For this review, take the finished solid that the model builds, in its own axes (mm). A direction names the side the tool comes from. Give positions to 0.01 mm unless a question says otherwise; leave off trailing zeros. Loops run counter-clockwise (first coordinate to the right, second up) from the corner with the lowest first, then second, coordinate; pieces in that order, holes last. Notation, with made-up numbers: (86.5, 85) - (126.5, 85) arc R11 cw to (126.5, 105) - close; hole circle Ø2 at (63.25, 42.25). An arc over 180 degrees is marked (long way). Answer in a Markdown table with one row per item.
```python
from build123d import *

# Parameters (mm, degrees)
SKETCH1_R               = 3.175
BOSS_EXTRUDE1_DEPTH     = 9.525
CUT_EXTRUDE1_DEPTH      = 6.35
CUT_EXTRUDE2_START      = -19.05
CUT_EXTRUDE2_DEPTH      = 6.35
BOSS_EXTRUDE2_DEPTH     = 6.35
CUT_EXTRUDE5_DEPTH      = 54.858594107
CUT_EXTRUDE5_DEPTH_BACK = 54.858594107


with BuildPart() as part:
    # Sketch1 → Boss-Extrude1 (new, symmetric)
    with BuildSketch(Plane.XY):
        with BuildLine():
            Line((6.300964517, 11.912379435), (50.8, 6.35))
            Line((50.8, 6.35), (7.193167088, 6.35))
            Line((7.193167088, 6.35), (6.300964517, -0.787620565))
            ThreePointArc((6.300964517, -0.787620565), (4.202446277, -4.760456416), (0, -6.35))
            ThreePointArc((0, -6.35), (-4.760456416, -4.202446277), (-6.300964517, 0.787620565))
            ThreePointArc((-6.300964517, 0.787620565), (-4.202446277, 4.760456416), (0, 6.35))
            Line((0, 6.35), (0.781538462, 12.602307692))
            Line((0.781538462, 12.602307692), (6.300964517, 11.912379435))
        make_face()
        with Locations(Location((0, 0, 0), (0, 0, 180))):
            Circle(SKETCH1_R, mode=Mode.SUBTRACT)
    extrude(amount=BOSS_EXTRUDE1_DEPTH, both=True)

    # Sketch2 → Cut-Extrude1 (cut)
    with BuildSketch(Plane.XY.offset(9.525)):
        Polygon((7.193167088, 21.115513253), (-6.35, 21.115513253), (-6.35, 0.257727368), (-6.35, -6.35), (7.193167088, -6.35), (7.193167088, 6.35), (8.941363703, 20.335572925), align=None)
    extrude(amount=-CUT_EXTRUDE1_DEPTH, mode=Mode.SUBTRACT)

    # Sketch2<2> → Cut-Extrude2 (cut)
    with BuildSketch(Plane.XY.offset(9.525).offset(CUT_EXTRUDE2_START)):
        Polygon((7.193167088, 21.115513253), (-6.35, 21.115513253), (-6.35, 0.257727368), (-6.35, -6.35), (7.193167088, -6.35), (7.193167088, 6.35), (8.941363703, 20.335572925), align=None)
    extrude(amount=CUT_EXTRUDE2_DEPTH, mode=Mode.SUBTRACT)

    # Sketch3 → Boss-Extrude2 (add)
    with BuildSketch(Plane.XY.offset(3.175)):
        with BuildLine():
            Line((-1.905, 2.54), (-1.905, -2.54))
            ThreePointArc((-1.905, -2.54), (-3.175, 0), (-1.905, 2.54))
        make_face()
    extrude(amount=-BOSS_EXTRUDE2_DEPTH)

    # Sketch4 → Cut-Extrude5 (cut, two sides: drawn at the far end of the back side and taken through both)
    with BuildSketch(Plane.XY.offset(3.175).offset(-CUT_EXTRUDE5_DEPTH_BACK)):
        with BuildLine():
            Line((0.787620565, 6.300964517), (1.563076923, 12.504615385))
            Line((1.563076923, 12.504615385), (-1.51572631, 12.889465789))
            Line((-1.51572631, 12.889465789), (-2.391608705, 5.882406634))
            ThreePointArc((-2.391608705, 5.882406634), (-0.828849904, 6.29567374), (0.787620565, 6.300964517))
        make_face()
    extrude(amount=CUT_EXTRUDE5_DEPTH + CUT_EXTRUDE5_DEPTH_BACK, mode=Mode.SUBTRACT)


solid = part.part
```
1. We need section A-A, the plane y = 0. Give the boundary of the cut face in (x, z) (3 decimals), and give its area (3 significant figures).
Values:
| item | result |
|---|---|
| outline | (-6.35, -3.175) - (-1.905, -3.175) - (-1.905, 3.175) - (-6.35, 3.175) - close; (3.175, -3.175) - (6.399, -3.175) - (6.399, 3.175) - (3.175, 3.175) - close |
| area | 48.7 mm^2 |
2. We need section B-B, the plane z = 1.5. Give the boundary of the cut face in (x, y) (3 decimals), and give its area (3 significant figures).
Values:
| item | result |
|---|---|
| outline | (0.788, 6.301) arc R6.35 ccw (long way) to (6.301, -0.788) - (7.193, 6.35) - (50.8, 6.35) - (1.563, 12.505) - close; hole (-1.905, -2.54) arc R3.175 ccw (long way) to (-1.905, 2.54) - close |
| area | 265 mm^2 |
3. Clearance check with flat-ended pins moving along their axes: pin 1 (3 mm diameter, centred on x = 28, z = -7.5, fed in from +Y); pin 2 (1 mm diameter, centred on y = 5.5, z = -1.5, fed in from +X); pin 3 (7 mm diameter, centred on x = -0.5, y = 1, fed in from -Z) (3 decimals); pin 4 (6 mm diameter, centred on x = 42.5, y = 0.5, fed in from +Z). State where each tip first meets the part, or that it passes through.
Values:
| item | result |
|---|---|
| pin 1 | stops at y = 9.39 |
| pin 2 | stops at x = 7.15 |
| pin 3 | stops at z = -3.175 |
| pin 4 | passes through |
4. Mouldability with a two-part tool opening along X and no side actions: class faces 1 (the face through (2, 3, 3.175)), 2 (the face through (-1.905, 0, 0)), 3 (the face through (7.524, 8.996, 6.394)), 4 (the face through (3.173, -0.098, -0.044)) as released by +X, released by -X, zero draft, split by the parting line, or undercut.
Values:
| item | result |
|---|---|
| face 1 | zero draft |
| face 2 | undercut |
| face 3 | released by -X |
| face 4 | undercut |
5. We need section D-D, the plane z = -7.5. Give the boundary of the cut face in (x, y), and give its area (3 significant figures).
Values:
| item | result |
|---|---|
| outline | (7.19, 6.35) - (50.8, 6.35) - (7.86, 11.72) - close |
| area | 117 mm^2 |
6. For faces 5 (the face through (7.524, 8.996, -6.394)), 6 (the face through (29, 6.35, 0)), 7 (the face through (20, 8, 9.525)), list the 3-axis set-ups (+Z, -Z, +X, -X, +Y, -Y) from which the entire face can be reached by the end or side of a thin tool; tool diameter is ignored.
Values:
| item | result |
|---|---|
| face 5 | -Z, -X, +Y |
| face 6 | +Z, -Z, +X, -Y |
| face 7 | +Z, +X, -X, +Y, -Y |
7. We need section C-C, the plane x = 32. Give the boundary of the cut face in (y, z) (3 decimals), and give its area (3 significant figures).
Values:
| item | result |
|---|---|
| outline | (6.35, -9.525) - (8.7, -9.525) - (8.7, 9.525) - (6.35, 9.525) - close |
| area | 44.8 mm^2 |
8. Wall thickness on line 1 (Z direction, x = 7, y = 6.5) (3 decimals); line 2 (Y direction, x = 36, z = -6.75); line 3 (X direction, y = 3.25, z = 1): over which ranges is each line inside the solid? List them lowest first. Write a range as [from, to].
Values:
| item | result |
|---|---|
| line 1 | z = [-3.175, 3.175] |
| line 2 | y = [6.35, 8.2] |
| line 3 | x = [-5.46, 6.81] |
